Source: three-view drawing plus pictorial views. Frame: mm from the lowest corner of the part. Coordinates: 2 decimals unless noted, no trailing zeros. Order: outer loops, then holes, each group sorted by start corner. A loop starts at its lowest first (then second) coordinate and runs counter-clockwise, first axis right, second up. Notation, with made-up numbers: (42, 64.25) - (90, 64.25) arc R28 ccw to (90, 102.25) - close; hole circle Ø4 at (-20, 76.25). An arc over 180 degrees is marked (long way). One line per question, with ' | ' between items.
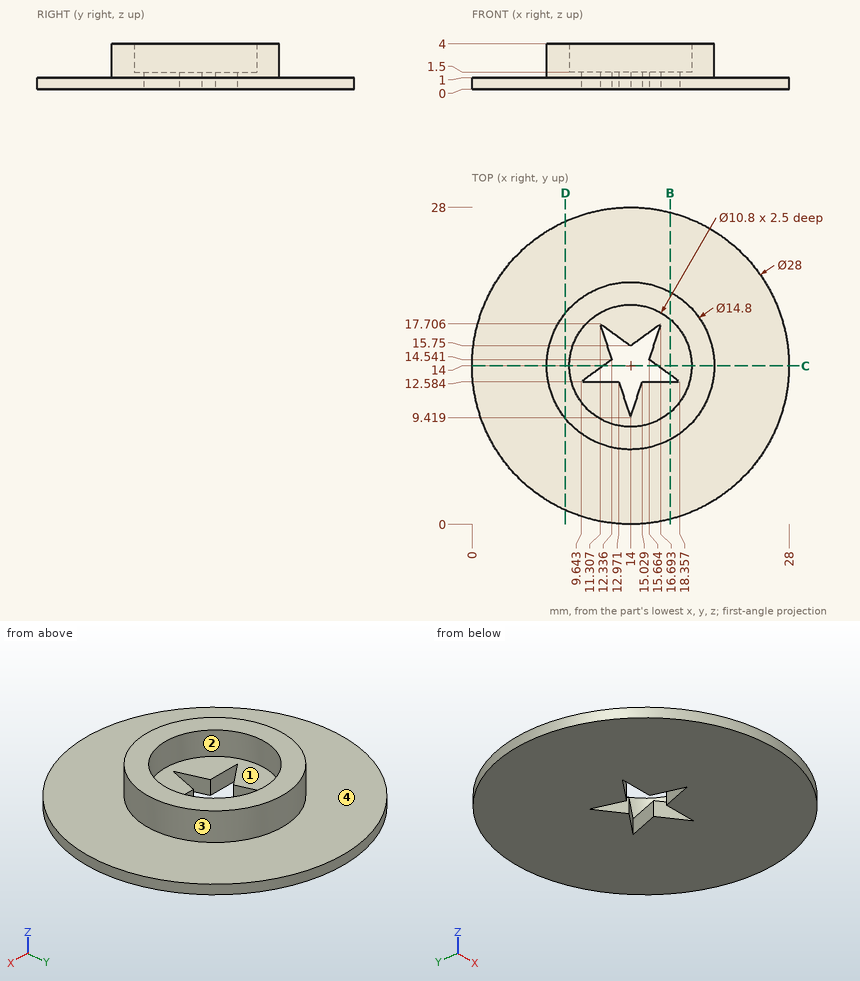
(1) Cut plane B-B (x = 17.5). Return the cut outline in (y, z) (1 decimal).
Taken from the geometry:
outline: (0.4, 0) - (12.6, 0) - (12.6, 1.5) - (9.9, 1.5) - (9.9, 4) - (7.5, 4) - (7.5, 1) - (0.4, 1) - close; (13.2, 0) - (27.6, 0) - (27.6, 1) - (20.5, 1) - (20.5, 4) - (18.1, 4) - (18.1, 1.5) - (13.2, 1.5) - close
(2) Material intervals for L1, parallel to X at y = 14, z = 2.3; L2, parallel to Z at x = 4, y = 20, sorted ascending. Write a range as from..to.
Taken from the geometry:
L1: x = 6.6..8.6, 19.4..21.4 | L2: z = 0..1
(3) Cut plane C-C (y = 14). Return the cut outline in (x, z).
Taken from the geometry:
outline: (0, 0) - (11.59, 0) - (11.59, 1.5) - (8.6, 1.5) - (8.6, 4) - (6.6, 4) - (6.6, 1) - (0, 1) - close; (16.41, 0) - (28, 0) - (28, 1) - (21.4, 1) - (21.4, 4) - (19.4, 4) - (19.4, 1.5) - (16.41, 1.5) - close
(4) Pin query (flat end, axial travel): P1, Ø2, axis at x = 15.5, z = 1, coming from the -Y side; P2, Ø1.5, axis at y = 8, z = 1, coming from the -X side; P3, Ø4, axis at x = 24, y = 11, coming from the +Z side. Return the tip coordinate at first contact, or that it passes through.
Taken from the geometry:
P1: stops at y = 0.01 | P2: stops at x = 1.02 | P3: stops at z = 1
(5) Pull-direction query (X, two-part tool) for the marked faces 1, 2, 3 and 4; classes: pulls with the +X half, pulls with the -X half, needs draft (parallel to the pull), parting line crosses it, or undercut.
Taken from the geometry:
face 1: undercut | face 2: undercut | face 3: parting line crosses it | face 4: needs draft
(6) Cut plane D-D (x = 8.25). Return the cut outline in (y, z) (1 decimal).
Taken from the geometry:
outline: (1.2, 0) - (26.8, 0) - (26.8, 1) - (18.7, 1) - (18.7, 4) - (9.3, 4) - (9.3, 1) - (1.2, 1) - close
